Can you work these out from the model? Positions are in its coordinate system, mm. A direction names the side the tool comes from. Give positions to 0.01 mm unless a question says otherwise; leave off trailing zeros. Loops run counter-clockwise (first coordinate to the right, second up) from the corner with the lowest first, then second, coordinate; pieces in that order, holes last. Notation, with made-up numbers: M 48,36.5 L 102,36.5 A4 ccw 102,41.5 Z; hole C -17.75,75 d9. An arc over 180 degrees is marked long. Put each result on its own line as item: value. Start each with the question number.
1) For faces 1 (the flat face through (-29.195, 6, -17)), 2 (the flat face through (0, 6, -14.3)), 3 (the flat face through (29.695, 6, -68)), which set-ups out of +Z, -Z, +X, -X, +Y, -Y let a thin tool reach every point of the face, with its end or its side?
2) Imagine slicing it at B-B (y = 8). State how many separate pieces and enclosed holes the cut face has, then the cut area to 3 significant figures.
3) For P1, Ø5, axis at y = 6.5, z = 19, coming from the -X side (3 decimals); P2, Ø1.5, axis at y = 5, z = 2, coming from the +X side (3 decimals); P3, Ø2.5, axis at x = -7.5, y = 5, coming from the -Z side, each with a flat end and sliding along its axis, tell me the tip position at first contact or that it passes through.
4) Imagine slicing it at A-A (z = -34.2). Write out the boundary of the cut face in (x, y) (3 decimals).
5) Imagine slicing it at D-D (z = 24.5). Write out the boundary of the cut face in (x, y).
6) Please list where these lines run through material, in increasing order: line 1 along X through (y, z) = (0.65, -68.4); line 2 along X through (y, z) = (8.75, -52) (3 decimals); line 3 along Y through (x, z) = (2.5, 21.5). Write a range as from..to.
7) If we mould it in two halves opening along X, with no side actions, what happens to faces 4 (the flat face through (0, 10.1, 68)), 5 (the cylindrical face through (44.364, 0.811, 0.215)), 6 (the cylindrical face through (44.61, 0.81, 67.51)), 7 (the flat face through (-29.195, 6, -34))? For each: +X half, -X half, draft (parallel to the pull), parting line (faces both ways), or undercut.
from build123d import *

# Parameters (mm, degrees)
SKETCH1_W           = 99.5
SKETCH1_H           = 146.8
BOSS_EXTRUDE1_DEPTH = 1.6
SKETCH3_R           = 1.65
CUT_EXTRUDE2_DEPTH  = 1.6
SKETCH4_W           = 58.89
SKETCH4_H           = 5.6
BOSS_EXTRUDE2_DEPTH = 8.5
FILLET2_R           = 2


with BuildPart() as part:
    # Sketch1 → Boss-Extrude1 (new body)
    with BuildSketch(Plane(origin=(0, 0, 0), x_dir=(1, 0, 0), z_dir=(0, 1, 0))):
        Rectangle(SKETCH1_W, SKETCH1_H)
    extrude(amount=BOSS_EXTRUDE1_DEPTH)

    # Sketch3 → Cut-Extrude2 (cut)
    with BuildSketch(Plane(origin=(0, 1.6, 0), x_dir=(1, 0, 0), z_dir=(0, 1, 0))):
        with Locations(Location((-46, -68.4, 0), (0, 0, 270))):
            Circle(SKETCH3_R)
        with Locations(Location((-46, -51.3, 0), (0, 0, 270))):
            Circle(SKETCH3_R)
        with Locations(Location((-46, -34.2, 0), (0, 0, 270))):
            Circle(SKETCH3_R)
        with Locations(Location((-46, -17.1, 0), (0, 0, 270))):
            Circle(SKETCH3_R)
        with Locations(Location((-46, 0, 0), (0, 0, 270))):
            Circle(SKETCH3_R)
        with Locations(Location((-46, 17.1, 0), (0, 0, 270))):
            Circle(SKETCH3_R)
        with Locations(Location((-46, 34.2, 0), (0, 0, 270))):
            Circle(SKETCH3_R)
        with Locations(Location((-46, 51.3, 0), (0, 0, 270))):
            Circle(SKETCH3_R)
        with Locations(Location((-46, 68.4, 0), (0, 0, 270))):
            Circle(SKETCH3_R)
        with Locations(Location((46, 68.4, 0), (0, 0, 90))):
            Circle(SKETCH3_R)
        with Locations(Location((46, 51.3, 0), (0, 0, 90))):
            Circle(SKETCH3_R)
        with Locations(Location((46, 34.2, 0), (0, 0, 90))):
            Circle(SKETCH3_R)
        with Locations(Location((46, 17.1, 0), (0, 0, 90))):
            Circle(SKETCH3_R)
        with Locations(Location((46, 0, 0), (0, 0, 90))):
            Circle(SKETCH3_R)
        with Locations(Location((46, -17.1, 0), (0, 0, 90))):
            Circle(SKETCH3_R)
        with Locations(Location((46, -34.2, 0), (0, 0, 90))):
            Circle(SKETCH3_R)
        with Locations(Location((46, -51.3, 0), (0, 0, 90))):
            Circle(SKETCH3_R)
        with Locations(Location((46, -68.4, 0), (0, 0, 90))):
            Circle(SKETCH3_R)
    extrude(amount=-CUT_EXTRUDE2_DEPTH, mode=Mode.SUBTRACT)

    # Sketch4 → Boss-Extrude2 (add)
    with BuildSketch(Plane(origin=(0, 1.6, 0), x_dir=(1, 0, 0), z_dir=(0, 1, 0))):
        with Locations((0.25, -51.3)):
            Rectangle(SKETCH4_W, SKETCH4_H)
        with Locations((0.25, -68.4)):
            Rectangle(SKETCH4_W, SKETCH4_H)
        with Locations((0.25, -34.2)):
            Rectangle(SKETCH4_W, SKETCH4_H)
        with Locations((0.25, -17.1)):
            Rectangle(SKETCH4_W, SKETCH4_H)
        with Locations((0.25, 0)):
            Rectangle(SKETCH4_W, SKETCH4_H)
        with Locations((0.25, 17.1)):
            Rectangle(SKETCH4_W, SKETCH4_H)
        with Locations((0.25, 34.2)):
            Rectangle(SKETCH4_W, SKETCH4_H)
        with Locations((0.25, 51.3)):
            Rectangle(SKETCH4_W, SKETCH4_H)
        with Locations((0.25, 68.4)):
            Rectangle(SKETCH4_W, SKETCH4_H)
    extrude(amount=BOSS_EXTRUDE2_DEPTH)

    # Fillet2
    fillet2_edges = [part.edges().sort_by_distance(p)[0] for p in [
        (49.75, 0.8, 73.4),
        (-49.75, 0.8, 73.4),
        (-49.75, 0.8, -73.4),
        (49.75, 0.8, -73.4),
    ]]
    fillet(fillet2_edges, radius=FILLET2_R)


solid = part.part
Recorded:
1. face 1: +Z, -Z, -X, +Y
1. face 2: +X, -X, +Y
1. face 3: +Z, -Z, +X, +Y
2. separate pieces: 9
2. enclosed holes: 0
2. area: 2,970 mm²
3. P1: x = -29.195
3. P2: x = 29.695
3. P3: z = -71.2
4. outline: M -49.75,0 L -47.65,0 L -47.65,1.6 L -49.75,1.6 Z; M -44.35,0 L 44.35,0 L 44.35,1.6 L 29.695,1.6 L 29.695,10.1 L -29.195,10.1 L -29.195,1.6 L -44.35,1.6 Z; M 47.65,0 L 49.75,0 L 49.75,1.6 L 47.65,1.6 Z
5. outline: M -49.75,0 L 49.75,0 L 49.75,1.6 L -49.75,1.6 Z
6. line 1: -49.75..-47.65, -44.35..44.35, 47.65..49.75
6. line 2: -29.195..29.695
6. line 3: 0..1.6
7. face 4: draft
7. face 5: undercut
7. face 6: undercut
7. face 7: -X half
